Part model, mm, in its own coordinate system. A direction names the side the tool comes from. Round coordinates to 2 decimals unless told otherwise and drop trailing zeros. Order: outer loops, then holes, each group sorted by start corner. A loop starts at its lowest first (then second) coordinate and runs counter-clockwise, first axis right, second up. Notation, with made-up numbers: (77.25, 50.5) - (118.25, 50.5) arc R19 cw to (118.25, 80.5) - close; hole circle Ø3 at (-13, 35). An arc over 180 degrees is marked (long way). Return JSON: item names as keys, results as strings. Group by question number.
Item 1: Tool access for faces 4 (the face through (-66, -19.05, 46)), 5 (the face through (-55.1, 0, 20.9)), 6 (the face through (-37, -13, 21.066)): list every direction of +Z, -Z, +X, -X, +Y, -Y with a clear straight run to the whole face (end or side of a thin tool).
Item 2: Saw through at B-B on x = -69. List the corners of the cut face in (y, z), and give its area (3 significant figures).
Item 3: Saw through at D-D on x = -25.5. List the corners of the cut face in (y, z).
Item 4: Saw through at A-A on z = 19.5. List the corners of the cut face in (x, y), and give its area (3 significant figures).
Item 5: Two-plate mould, pull along Y, no slides. Class faces 1 (the face through (-72.086, -13, 25)), 2 (the face through (-55.1, -25.4, 20.9)), 3 (the face through (-24.706, -18.334, 14.805)): released by +Y, released by -Y, zero draft, split by the parting line, or undercut.
Item 6: Drop flat-ended pins along their axis: pin 1 (5 mm diameter, centred on x = -29.5, y = -17, fed in from +Z); pin 2 (2 mm diameter, centred on y = -11, z = 23.5, fed in from +X); pin 3 (9 mm diameter, centred on x = -68.5, z = 46.5, fed in from -Y); pin 4 (11.5 mm diameter, centred on x = -46.69, y = -12.7, fed in from +Z). Give the stop position or say it passes through.
Item 7: Probe probe 1 along X at (y, z) = (-11, 19); probe 2 along X at (y, z) = (-12.25, 17); probe 3 along X at (y, z) = (-5.25, 34). List the from-to ranges inside material, lowest first.
Item 8: Saw through at C-C on y = -17. List the corners of the cut face in (x, z).
```python
from build123d import *

# Parameters (mm, degrees)
F1_DEPTH = 25.4
F2_R     = 6.35
F3_DEPTH = 12.701
F5_DEPTH = 12.701
F7_DEPTH = 12.701
F9_DEPTH = 12.701


with BuildPart() as f1:
    # F0 (on Front) → F1 (new body)
    with BuildSketch(Plane.XZ):
        Polygon((-72.08584, 8.36633), (-14.93584, 8.36633), (-14.93584, 21.06633), (-59.38584, 21.06633), (-59.38584, 52.81633), (-72.08584, 52.81633), align=None)
    extrude(amount=F1_DEPTH)

    # F2 (on face) → F3 (cut, through all)
    with BuildSketch(Plane.XY.offset(21.06633)):
        with Locations((-46.68584, -12.7)):
            Circle(F2_R)
        with Locations((-27.63584, -12.7)):
            Circle(F2_R)
    extrude(amount=-F3_DEPTH, mode=Mode.SUBTRACT)

    # F4 (on face) → F5 (cut, through all)
    with BuildSketch(Plane.XY.offset(21.06633)):
        with BuildLine():
            ThreePointArc((-27.63584, 0), (-18.655584, -3.719744), (-14.93584, -12.7))
            Line((-14.93584, -12.7), (-14.93584, 0))
            Line((-14.93584, 0), (-27.63584, 0))
        make_face()
        with BuildLine():
            ThreePointArc((-14.93584, -12.7), (-18.655584, -21.680256), (-27.63584, -25.4))
            Line((-27.63584, -25.4), (-14.93584, -25.4))
            Line((-14.93584, -25.4), (-14.93584, -12.7))
        make_face()
    extrude(amount=-F5_DEPTH, mode=Mode.SUBTRACT)

    # F6 (on face) → F7 (cut, through all)
    with BuildSketch(Plane.YZ.offset(-59.38584)):
        with BuildLine():
            ThreePointArc((-25.4, 40.11633), (-21.680256, 49.096586), (-12.7, 52.81633))
            Line((-12.7, 52.81633), (-25.4, 52.81633))
            Line((-25.4, 52.81633), (-25.4, 40.11633))
        make_face()
        with BuildLine():
            ThreePointArc((-12.7, 52.81633), (-3.719744, 49.096586), (0, 40.11633))
            Line((0, 40.11633), (0, 52.81633))
            Line((0, 52.81633), (-12.7, 52.81633))
        make_face()
    extrude(amount=-F7_DEPTH, mode=Mode.SUBTRACT)

    # F8 (on face) → F9 (cut, through all)
    with BuildSketch(Plane.YZ.offset(-59.38584)):
        with BuildLine():
            ThreePointArc((-19.05, 40.11633), (-12.7, 33.76633), (-6.35, 40.11633))
            Line((-6.35, 40.11633), (-12.7, 40.11633))
            Line((-12.7, 40.11633), (-19.05, 40.11633))
        make_face()
        with BuildLine():
            ThreePointArc((-19.05, 40.11633), (-12.7, 46.46633), (-6.35, 40.11633))
            Line((-6.35, 40.11633), (-6.35, 51.114853))
            ThreePointArc((-6.35, 51.114853), (-12.7, 52.81633), (-19.05, 51.114853))
            Line((-19.05, 51.114853), (-19.05, 40.11633))
        make_face()
        with BuildLine():
            Line((-12.7, 40.11633), (-6.35, 40.11633))
            ThreePointArc((-6.35, 40.11633), (-12.7, 46.46633), (-19.05, 40.11633))
            Line((-19.05, 40.11633), (-12.7, 40.11633))
        make_face()
    extrude(amount=-F9_DEPTH, mode=Mode.SUBTRACT)


solid = f1.part
```
Filled in:
{
 "1": {"face 4": "+Z, +X, -X", "face 5": "+Z, -Z, +X, -X, +Y", "face 6": "+Z, +X, +Y, -Y"},
 "2": {"outline": "(-25.4, 8.37) - (0, 8.37) - (0, 40.12) arc R12.7 ccw to (-6.35, 51.11) - (-6.35, 40.12) arc R6.35 cw to (-19.05, 40.12) - (-19.05, 51.11) arc R12.7 ccw to (-25.4, 40.12) - close", "area": "842 mm^2"},
 "3": {"outline": "(-25.22, 8.37) - (-18.68, 8.37) - (-18.68, 21.07) - (-25.22, 21.07) - close; (-6.72, 8.37) - (-0.18, 8.37) - (-0.18, 21.07) - (-6.72, 21.07) - close"},
 "4": {"outline": "(-72.09, -25.4) - (-27.64, -25.4) arc R12.7 ccw to (-27.64, 0) - (-72.09, 0) - close; hole circle Ø12.7 at (-46.69, -12.7); hole circle Ø12.7 at (-27.64, -12.7)", "area": "1,130 mm^2"},
 "5": {"face 1": "zero draft", "face 2": "released by -Y", "face 3": "undercut"},
 "6": {"pin 1": "stops at z = 21.07", "pin 2": "stops at x = -59.39", "pin 3": "stops at y = -25.26", "pin 4": "passes through"},
 "7": {"probe 1": "x = -72.09 to -52.8, -40.57 to -33.75, -21.52 to -15.05", "probe 2": "x = -72.09 to -53.02, -40.35 to -33.97, -21.3 to -14.94", "probe 3": "x = -72.09 to -59.39"},
 "8": {"outline": "(-72.09, 8.37) - (-51.36, 8.37) - (-51.36, 21.07) - (-59.39, 21.07) - (-59.39, 35.44) - (-72.09, 35.44) - close; (-42.01, 8.37) - (-32.31, 8.37) - (-32.31, 21.07) - (-42.01, 21.07) - close; (-22.96, 8.37) - (-15.69, 8.37) - (-15.69, 21.07) - (-22.96, 21.07) - close"}
}
